Geometry: see drawing. Coordinates: mm, zero at the bounding-box minimum. Round coordinates to 2 decimals unless told otherwise and drop trailing zeros. Loops run counter-clockwise (first coordinate to the right, second up) from the corner with the lowest first, then second, coordinate; pieces in that order, holes last.
(1) First-contact query: pin 1 Ø8 at (y, z) = (48, 15) entering from -X; pin 2 Ø0.9 at (x, y) = (1, 74) entering from -Z; pin 3 Ø1.5 at (x, z) = (1.5, 88.5) entering from -Y; pin 4 Ø1.5 at (x, z) = (1, 89.5) entering from +Y. Flat tips, straight axial feed; report the tip coordinate or a pass-through.
(2) Section B-B, the plane y = 56.5. Return the cut outline in (x, z).
(3) Section C-C, the plane z = 58.5. Return the cut outline in (x, y).
(4) Material intervals for probe 1 along Y at (x, z) = (2.2, 40); probe 2 along Z at (x, y) = (0.35, 22.5), sorted ascending.
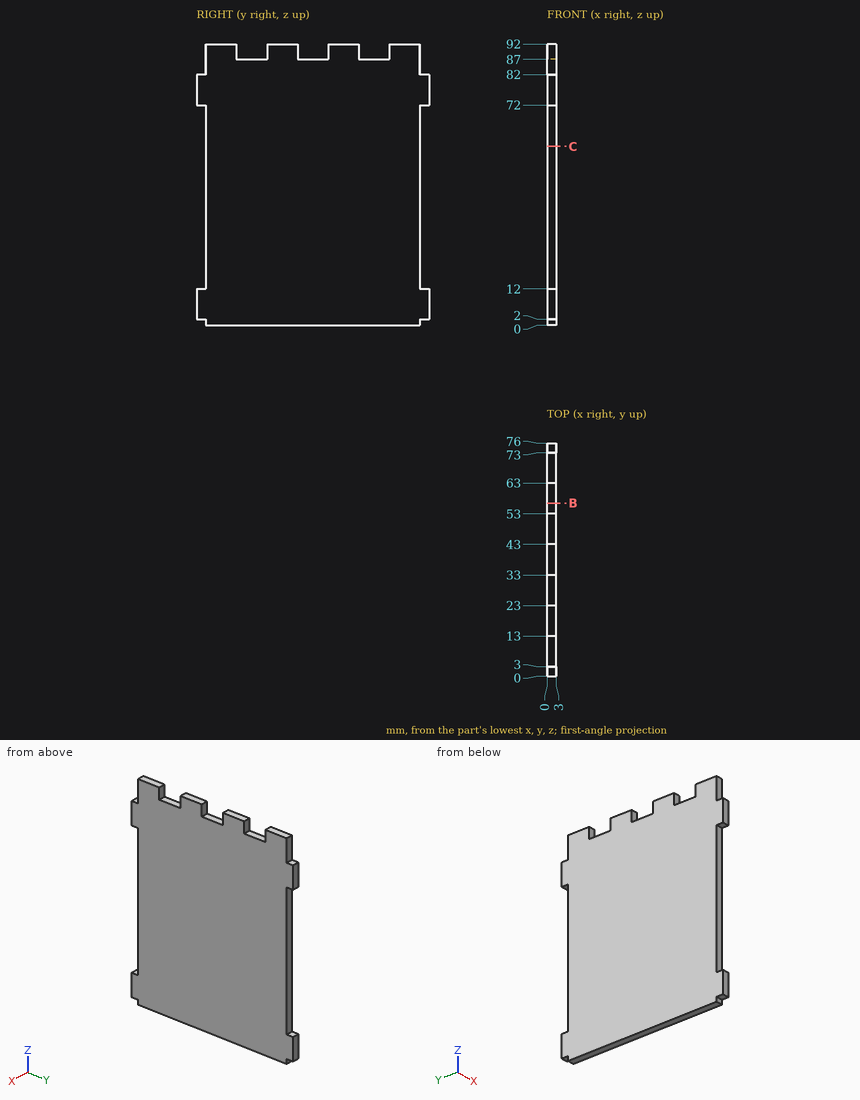
Output values:
1. pin 1: stops at x = 0
1. pin 2: stops at z = 2
1. pin 3: stops at y = 3
1. pin 4: stops at y = 73
2. outline: (0, 0) - (3, 0) - (3, 87) - (0, 87) - close
3. outline: (0, 3) - (3, 3) - (3, 73) - (0, 73) - close
4. probe 1: y = 3 to 73
4. probe 2: z = 0 to 87
